from build123d import *

# Parameters (mm, degrees)
BOSS_EXTRUDE1_DEPTH = 3.175
CUT_EXTRUDE2_START  = -3.175
CUT_EXTRUDE2_DEPTH  = 3.175
FILLET1_R           = 6
BOSS_EXTRUDE2_DEPTH = 3.175
SKETCH2_R           = 3
BOSS_EXTRUDE3_DEPTH = 6.35


with BuildPart() as part:
    # Sketch1 → Boss-Extrude1 (new body)
    with BuildSketch(Plane.XY):
        with BuildLine():
            Line((-32.352380638, 120.740728286), (0, 0))
            Line((0, 0), (0, 125))
            ThreePointArc((0, 125), (-16.315774028, 123.930607672), (-32.352380638, 120.740728286))
        make_face()
        with BuildLine():
            Line((0, 125), (0, 0))
            Line((0, 0), (32.352380638, 120.740728286))
            ThreePointArc((32.352380638, 120.740728286), (16.315774028, 123.930607672), (0, 125))
        make_face()
    extrude(amount=BOSS_EXTRUDE1_DEPTH)

    # Sketch3 → Cut-Extrude2 (cut)
    with BuildSketch(Plane.XY.offset(3.175).offset(CUT_EXTRUDE2_START)):
        with BuildLine():
            ThreePointArc((-12.5, 124.373429638), (-199.821294039, -6.943966706), (0, -118.321595662))
            ThreePointArc((0, -118.321595662), (-69.003341725, -16.373894052), (-26.577702514, 99.189336132))
            Line((-26.577702514, 99.189336132), (-32.352380638, 120.740728286))
            ThreePointArc((-32.352380638, 120.740728286), (-22.499625375, 122.958394825), (-12.5, 124.373429638))
        make_face()
        with BuildLine():
            ThreePointArc((-26.577702514, 99.189336132), (-13.871129508, 109.564341508), (0, 118.321595662))
            ThreePointArc((0, 118.321595662), (-6.172126729, 121.50835908), (-12.5, 124.373429638))
            ThreePointArc((-12.5, 124.373429638), (-22.499625375, 122.958394825), (-32.352380638, 120.740728286))
            Line((-32.352380638, 120.740728286), (-26.577702514, 99.189336132))
        make_face()
        with BuildLine():
            ThreePointArc((-12.5, 124.373429638), (-6.172126729, 121.50835908), (0, 118.321595662))
            ThreePointArc((0, 118.321595662), (6.172126729, 121.50835908), (12.5, 124.373429638))
            ThreePointArc((12.5, 124.373429638), (0, 125), (-12.5, 124.373429638))
        make_face()
        with BuildLine():
            ThreePointArc((26.577702514, 99.189336132), (58.668892288, 54.138757654), (70, 0))
            ThreePointArc((70, 0), (51.189500386, -68.738635424), (0, -118.321595662))
            ThreePointArc((0, -118.321595662), (133.738635424, -116.189500386), (200, 0))
            ThreePointArc((200, 0), (139.624057783, 112.5), (12.5, 124.373429638))
            ThreePointArc((12.5, 124.373429638), (22.499625375, 122.958394825), (32.352380638, 120.740728286))
            Line((32.352380638, 120.740728286), (26.577702514, 99.189336132))
        make_face()
        with BuildLine():
            ThreePointArc((0, 118.321595662), (13.871129508, 109.564341508), (26.577702514, 99.189336132))
            Line((26.577702514, 99.189336132), (32.352380638, 120.740728286))
            ThreePointArc((32.352380638, 120.740728286), (22.499625375, 122.958394825), (12.5, 124.373429638))
            ThreePointArc((12.5, 124.373429638), (6.172126729, 121.50835908), (0, 118.321595662))
        make_face()
    extrude(amount=CUT_EXTRUDE2_DEPTH, mode=Mode.SUBTRACT)

    # Fillet1
    fillet1_edges = [part.edges().sort_by_distance(p)[0] for p in [
        (0, 118.321595662, 1.5875),
        (-26.577702514, 99.189336132, 1.5875),
        (26.577702514, 99.189336132, 1.5875),
    ]]
    fillet(fillet1_edges, radius=FILLET1_R)

    # Sketch4 → Boss-Extrude2 (add)
    with BuildSketch(Plane.XY.offset(3.175)):
        with BuildLine():
            Line((7, 101), (-7, 101))
            ThreePointArc((-7, 101), (-9, 103), (-7, 105))
            Line((-7, 105), (7, 105))
            ThreePointArc((7, 105), (9, 103), (7, 101))
        make_face()
    extrude(amount=BOSS_EXTRUDE2_DEPTH)

    # Sketch2 → Boss-Extrude3 (add)
    with BuildSketch(Plane.XY.offset(3.175)):
        with Locations((0, 108.5)):
            Circle(SKETCH2_R)
    extrude(amount=BOSS_EXTRUDE3_DEPTH)


solid = part.part
Design review of the part built by this model. Coordinates are the model's own, in mm. A direction names the side the tool comes from. Round coordinates to 2 decimals unless told otherwise and drop trailing zeros. Loops run counter-clockwise (first coordinate to the right, second up) from the corner with the lowest first, then second, coordinate; pieces in that order, holes last. Notation, with made-up numbers: (73.5, -26) - (90.5, -26) arc R3 cw to (90.5, -21) - close; hole circle Ø3 at (9, 34). An arc over 180 degrees is marked (long way). One line per item, written item: value. Start each with the question number.
1) To check wall thickness, follow L1, parallel to Z at x = 17, y = 96 (3 decimals); L2, parallel to Y at x = 2, z = 8.25; L3, parallel to X at y = 36.5, z = 2.5. State the ranges of each line that lie inside material, in increasing order. Write a range as from..to.
2) Draft analysis for pull direction Y (two halves, no side actions). For faces 4 (the cylindrical face through (-0.65, 105.57, 6.31)), 5 (the flat face through (0, 73, 0)), 6 (the flat face through (-12.992, 48.486, 1.565)), 7 (the cylindrical face through (9, 103, 5)), state which applies: +Y half, -Y half, draft (parallel to the pull), parting line (faces both ways), or undercut.
3) Consider section A-A on x = -5.5. Give the boundary of the cut face in (y, z) (3 decimals).
4) Consider section D-D on y = 78. Give the boundary of the cut face in (x, z) (3 decimals), then the cut area to 3 significant figures.
5) For faces 1 (the cylindrical face through (-9, 103, 5)), 2 (the flat face through (0, 105, 5)), 3 (the flat face through (0, 101, 5)), list the 3-axis set-ups (+Z, -Z, +X, -X, +Y, -Y) from which the entire face can be reached by the end or side of a thin tool; tool diameter is ignored.
6) Insertion check: pin 1 Ø4 at (x, y) = (2.5, 64.5) entering from +Z (3 decimals); pin 2 Ø1 at (x, z) = (-1.5, 4) entering from -Y; pin 3 Ø2.5 at (x, z) = (-1.5, 4) entering from +Y. Each pin has a flat end and moves straight along its axis. Give the tip position at first contact, or say it passes through.
7) Consider section B-B on y = 103. Give the boundary of the cut face in (x, z) (3 decimals).
8) Consider section C-C on x = -13. Give the boundary of the cut face in (y, z) (3 decimals), then the cut area to 3 significant figures.
Reported:
1. L1: z = 0..3.175
1. L2: y = 106.26..110.74
1. L3: x = -9.78..9.78
2. face 4: undercut
2. face 5: draft
2. face 6: -Y half
2. face 7: parting line
3. outline: (20.526, 0) - (115.129, 0) - (115.129, 3.175) - (105, 3.175) - (105, 6.35) - (101, 6.35) - (101, 3.175) - (20.526, 3.175) - close
4. outline: (-20.9, 0) - (20.9, 0) - (20.9, 3.175) - (-20.9, 3.175) - close
4. area: 133 mm^2
5. face 1: +Z, -X
5. face 2: +Z, +X, -X
5. face 3: +Z, +X, -X, -Y
6. pin 1: stops at z = 3.175
6. pin 2: stops at y = 101
6. pin 3: stops at y = 117.4
7. outline: (-22.27, 0) - (22.27, 0) - (22.27, 3.175) - (9, 3.175) - (9, 6.35) - (-9, 6.35) - (-9, 3.175) - (-22.27, 3.175) - close
8. outline: (48.517, 0) - (110.186, 0) - (110.186, 3.175) - (48.517, 3.175) - close
8. area: 196 mm^2
